Design review of the part built by this model. Coordinates are the model's own, in mm. Face numbers are marked on the shaded views. A direction names the side the tool comes from. Give positions to 0.01 mm unless a question says otherwise; leave off trailing zeros. Order: outer loops, then holes, each group sorted by start corner. A loop starts at its lowest first (then second) coordinate and runs counter-clockwise, first axis right, second up. Notation, with made-up numbers: (14, 14) -> (50, 14) arc R15 cw to (50, 24) -> close; hole circle Ø7 at (-2.75, 48). An arc over 180 degrees is marked (long way). One line per item, written item: value.
Autodesk Inventor part; units mm, degrees
ref_plane "YZ Plane" through (0, 0, 0) normal (1, 0, 0) x (0, 1, 0)
ref_plane "XZ Plane" through (0, 0, 0) normal (0, 1, 0) x (-1, 0, 0)
ref_plane "XY Plane" through (0, 0, 0) normal (0, 0, 1) x (1, 0, 0)
sketch "Sketch1" plane through (0, 0, 0) normal (0, 0, 1) x (1, 0, 0)
  line L0 (-30, -30) -> (30, -30)
  line L1 (30, -30) -> (30, 30)
  line L2 (30, 30) -> (-30, 30)
  line L3 (-30, 30) -> (-30, -30)
  line L4 (-30, -30) -> (30, 30) construction
  line L5 (30, -30) -> (-30, 30) construction
  line L6 (30, 30) -> (25, 30) construction
  line L7 (25, 30) -> (25, 25) construction
  line L8 (-30, 30) -> (-25, 30) construction
  line L9 (-25, 30) -> (-25, 25) construction
  line L10 (-30, -30) -> (-30, -25) construction
  line L11 (-30, -25) -> (-25, -25) construction
  line L12 (30, -30) -> (30, -25) construction
  line L13 (30, -25) -> (25, -25) construction
  circle A0 centre (-25, 25) radius 1.5
  circle A1 centre (25, 25) radius 1.5
  circle A2 centre (25, -25) radius 1.5
  circle A3 centre (-25, -25) radius 1.5
  point P0 (0, 0)
  dimension "d0" = 60
  dimension "d1" = 60
  dimension "d2" = 5
  dimension "d3" = 5
  dimension "d4" = 5
  dimension "d5" = 5
  dimension "d6" = 5
  dimension "d7" = 5
  dimension "d8" = 5
  dimension "d9" = 5
  dimension "d10" = 3
  dimension "d11" = 3
  dimension "d12" = 3
  dimension "d13" = 3
extrude "Block" add sketch "Sketch1" along normal blind 60
sketch "Sketch2" plane through (30, -30, 0) normal (1, 0, 0) x (0, 0, -1)
  line L0 (0, 0) -> (0, 60) construction
  line L1 (-60, 0) -> (0, 60) construction
  circle A0 centre (-30, 30) radius 2.5
  point P0 (0, 30)
  dimension "d17" = 5
extrude "Motor Mount" cut sketch "Sketch2" against normal blind 60
sketch "Sketch3" plane through (30, -30, 0) normal (1, 0, 0) x (0, 0, -1)
  line L0 (0, 60) -> (-60, 60) construction
  line L1 (-60, 60) -> (-60, 50) construction
  line L2 (-60, 60) -> (-60, 0) construction
  line L3 (-60, 50) -> (0, 50) construction
  line L4 (0, 60) -> (0, 0) construction
  line L5 (-60, 0) -> (-60, 10) construction
  line L6 (-60, 10) -> (0, 10) construction
  circle A0 centre (-30, 30) radius 2.5 construction
  line L7 (-30, 30) -> (-25, 30) construction
  line L8 (-30, 30) -> (-35, 30) construction
  line L9 (-35, 30) -> (-35, 10) construction
  line L10 (-25, 30) -> (-25, 10) construction
  line L11 (-25, 30) -> (-25, 50) construction
  line L12 (-35, 30) -> (-35, 50) construction
  line L13 (-60, 50) -> (-35, 50)
  line L14 (-35, 10) -> (-60, 10)
  line L15 (-35, 10) -> (-35, 50)
  line L16 (-25, 50) -> (-25, 10)
  line L17 (0, 10) -> (-25, 10)
  line L18 (-25, 50) -> (0, 50)
  line L19 (0, 50) -> (0, 10)
  line L20 (-60, 10) -> (-60, 50)
  point P0 (0, 30)
  dimension "d20" = 10
  dimension "d21" = 10
  dimension "d22" = 5
  dimension "d23" = 5
extrude "Plastic Savings" cut sketch "Sketch3" against normal blind 60
fillet "Fillets FTW" radius 3 12 edges at (0, -30, 60) (0, -20, 60) (0, 30, 60) (0, 20, 60) (0, 20, 35) (0, -20, 35) (0, -20, 0) (0, -30, 0) (0, -20, 25) (0, 20, 25) (0, 30, 0) (0, 20, 0)
sketch "Sketch4" plane through (30, -17, 35) normal (0, 0, 1) x (1, 0, 0)
  line L0 (0, 19.5) -> (0, 14.5) construction
  line L1 (0, 17) -> (-4, 17) construction
  circle A0 centre (-4, 17) radius 1.5
  point P0 (-30, 17)
  dimension "d27" = 4
  dimension "d28" = 3
extrude "Axle Lock" cut sketch "Sketch4" against normal blind 3.75
properties part number "60x60Idler"
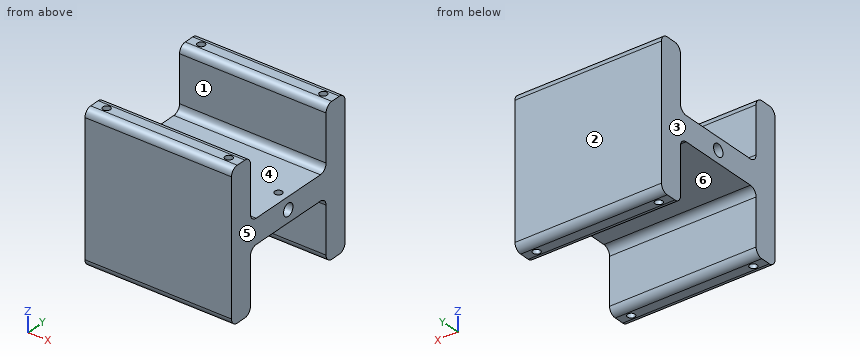
Item 1: Add section B-B on y = -25. Give the boundary of the cut face in (x, z), plus the area to 3 significant figures.
Returned:
outline: (-30, 0) -> (-26.5, 0) -> (-26.5, 60) -> (-30, 60) -> close; (-23.5, 0) -> (23.5, 0) -> (23.5, 60) -> (-23.5, 60) -> close; (26.5, 0) -> (30, 0) -> (30, 60) -> (26.5, 60) -> close
area: 3,240 mm²
Item 2: Machinability: for the marked faces 4, 5 and 6, which of the approach directions +Z, -Z, +X, -X, +Y, -Y give a long, thin tool a straight path to every point of the face, cutting with its end or side? Answer none if there is none.
Returned:
face 4: +Z, +X, -X
face 5: +Z, -Z, +X, +Y, -Y
face 6: -Z, +X, -X
Item 3: Add section D-D on z = 8.5. Give the boundary of the cut face in (x, y).
Returned:
outline: (-30, -30) -> (30, -30) -> (30, -20) -> (-30, -20) -> close; (-30, 20) -> (30, 20) -> (30, 30) -> (-30, 30) -> close; hole circle Ø3 at (-25, -25); hole circle Ø3 at (-25, 25); hole circle Ø3 at (25, -25); hole circle Ø3 at (25, 25)
Item 4: Draft analysis for pull direction Y (two halves, no side actions). For the marked faces 1, 2 and 3, state which applies: pulls with the +Y half, pulls with the -Y half, needs draft (parallel to the pull), parting line crosses it, or undercut.
Returned:
face 1: undercut
face 2: pulls with the +Y half
face 3: needs draft
Item 5: To check wall thickness, follow line 1 along Y through (x, z) = (25, 15); line 2 along Z through (x, y) = (10, 0); line 3 along Y through (x, z) = (-16, 57). State the ranges of each line that lie inside material, in increasing order. Write a range as from..to.
Returned:
line 1: -30..-26.5, -23.5..-20, 20..23.5, 26.5..30
line 2: 25..27.5, 32.5..35
line 3: -30..-20, 20..30
Item 6: Clearance check with flat-ended pins moving along their axes: P1, Ø17, axis at x = 9, y = 4.5, coming from the +Z side; P2, Ø1.8, axis at x = 25, y = -25, coming from the +Z side; P3, Ø5, axis at x = 26, y = 0, coming from the -Z side. State where each tip first meets the part, or that it passes through.
Returned:
P1: z = 35
P2: through
P3: z = 25
Item 7: Add section A-A on z = 30. Give the boundary of the cut face in (x, y), plus the area to 3 significant figures.
Returned:
outline: (-30, -30) -> (30, -30) -> (30, -2.5) -> (-30, -2.5) -> close; (-30, 2.5) -> (30, 2.5) -> (30, 30) -> (-30, 30) -> close; hole circle Ø3 at (-25, -25); hole circle Ø3 at (-25, 25); hole circle Ø3 at (25, -25); hole circle Ø3 at (25, 25)
area: 3,270 mm²
Item 8: Add section C-C on x = -21.5. Give the boundary of the cut face in (y, z).
Returned:
outline: (-30, 3) arc R3 ccw to (-27, 0) -> (-23, 0) arc R3 ccw to (-20, 3) -> (-20, 22) arc R3 cw to (-17, 25) -> (17, 25) arc R3 cw to (20, 22) -> (20, 3) arc R3 ccw to (23, 0) -> (27, 0) arc R3 ccw to (30, 3) -> (30, 57) arc R3 ccw to (27, 60) -> (23, 60) arc R3 ccw to (20, 57) -> (20, 38) arc R3 cw to (17, 35) -> (-17, 35) arc R3 cw to (-20, 38) -> (-20, 57) arc R3 ccw to (-23, 60) -> (-27, 60) arc R3 ccw to (-30, 57) -> close; hole circle Ø5 at (0, 30)
